Read the model definition and answer for the solid it produces. Units are mm, in the model's axes. Face numbers are marked on the shaded views. Round coordinates to 2 decimals unless told otherwise and drop trailing zeros. Loops run counter-clockwise (first coordinate to the right, second up) from the corner with the lowest first, then second, coordinate; pieces in that order, holes last. Notation, with made-up numbers: (-32.75, -35.75) - (-8.75, -35.75) arc R9 cw to (-8.75, -29.75) - close; hole circle Ø5 at (-22.5, 31). An arc over 180 degrees is marked (long way). Use one line per item in the form item = value. Start each with the question number.
```python
from build123d import *

# Parameters (mm, degrees)
F0_W     = 127
F0_H     = 127
F1_DEPTH = 12.7
F2_T     = -7.62
F4_DEPTH = 63.5


with BuildPart() as f1:
    # F0 (on Top) → F1 (new body)
    with BuildSketch(Plane.XY):
        Rectangle(F0_W, F0_H)
    extrude(amount=F1_DEPTH)

    # F2
    f2_openings = [f1.faces().sort_by_distance(p)[0] for p in [
        (0, 0, 12.7),
    ]]
    offset(amount=F2_T, openings=f2_openings)

    # F3 (on Front) → F4 (join, symmetric)
    with BuildSketch(Plane.XZ):
        Polygon((-63.5, 4.947344), (-65.025825, 4.947344), (-65.025825, 2.672656), (-63.5, 2.672656), (-63.5, 3.81), align=None)
        Polygon((-65.025825, 2.672656), (-65.025825, 4.947344), (-65.025825, 6.35), (-66.295825, 6.35), (-66.295825, 1.27), (-65.025825, 1.27), align=None)
        Polygon((65.025825, 6.35), (65.025825, 4.947344), (65.025825, 2.672656), (65.025825, 1.27), (66.295825, 1.27), (66.295825, 6.35), align=None)
        Polygon((65.025825, 2.672656), (65.025825, 4.947344), (63.5, 4.947344), (63.5, 3.81), (63.5, 2.672656), align=None)
    extrude(amount=F4_DEPTH, both=True)


solid = f1.part
```
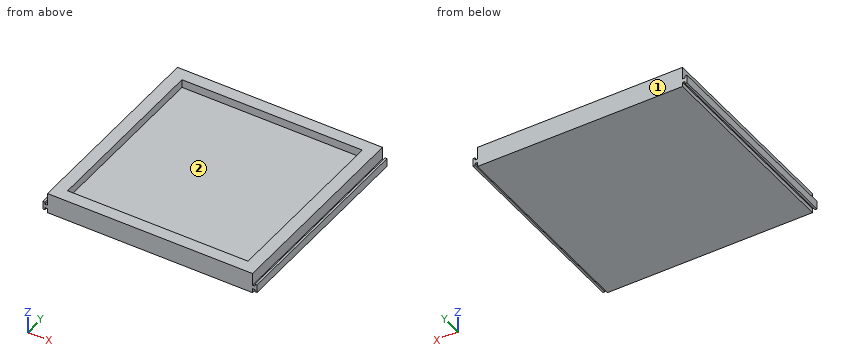
1) A cutting plane is placed at A-A on y = 46.5. Write down the section's boundary in (x, z), plus the area to 3 significant figures.
2) Determine the mould class of the marked faces 1 and 2 for opening direction X: +X half, -X half, draft (parallel to the pull), parting line (faces both ways), or undercut.
3) A cutting plane is placed at B-B on x = 35. Write down the section's boundary in (y, z), plus the area to 3 significant figures.
4) Straight lines are drawn through the part: line 1 (X direction, y = -28, z = 5.25); line 2 (X direction, y = 23.5, z = 11.25). For each, find the intervals that lie inside material, in ascending order. Write a range as from..to.
5) Flat-ended cylindrical pins translate along their axes: pin 1 (4 mm diameter, centred on x = -50.5, y = -33, fed in from +Z); pin 2 (0.5 mm diameter, centred on x = -64.5, y = 6, fed in from -Z); pin 3 (2 mm diameter, centred on y = -33.5, z = 8, fed in from +X). Find the tip coordinate at first contact, or state that the pin passes through.
Checks:
q1.outline = (-66.3, 1.27) - (-65.03, 1.27) - (-65.03, 2.67) - (-63.5, 2.67) - (-63.5, 0) - (63.5, 0) - (63.5, 2.67) - (65.03, 2.67) - (65.03, 1.27) - (66.3, 1.27) - (66.3, 6.35) - (65.03, 6.35) - (65.03, 4.95) - (63.5, 4.95) - (63.5, 12.7) - (55.88, 12.7) - (55.88, 7.62) - (-55.88, 7.62) - (-55.88, 12.7) - (-63.5, 12.7) - (-63.5, 4.95) - (-65.03, 4.95) - (-65.03, 6.35) - (-66.3, 6.35) - close
q1.area = 1,070 mm²
q2.face_1 = draft
q2.face_2 = undercut
q3.outline = (-63.5, 0) - (63.5, 0) - (63.5, 12.7) - (55.88, 12.7) - (55.88, 7.62) - (-55.88, 7.62) - (-55.88, 12.7) - (-63.5, 12.7) - close
q3.area = 1,050 mm²
q4.line_1 = -66.3..-65.03, -63.5..63.5, 65.03..66.3
q4.line_2 = -63.5..-55.88, 55.88..63.5
q5.pin_1 = 7.62
q5.pin_2 = 2.67
q5.pin_3 = 63.5
